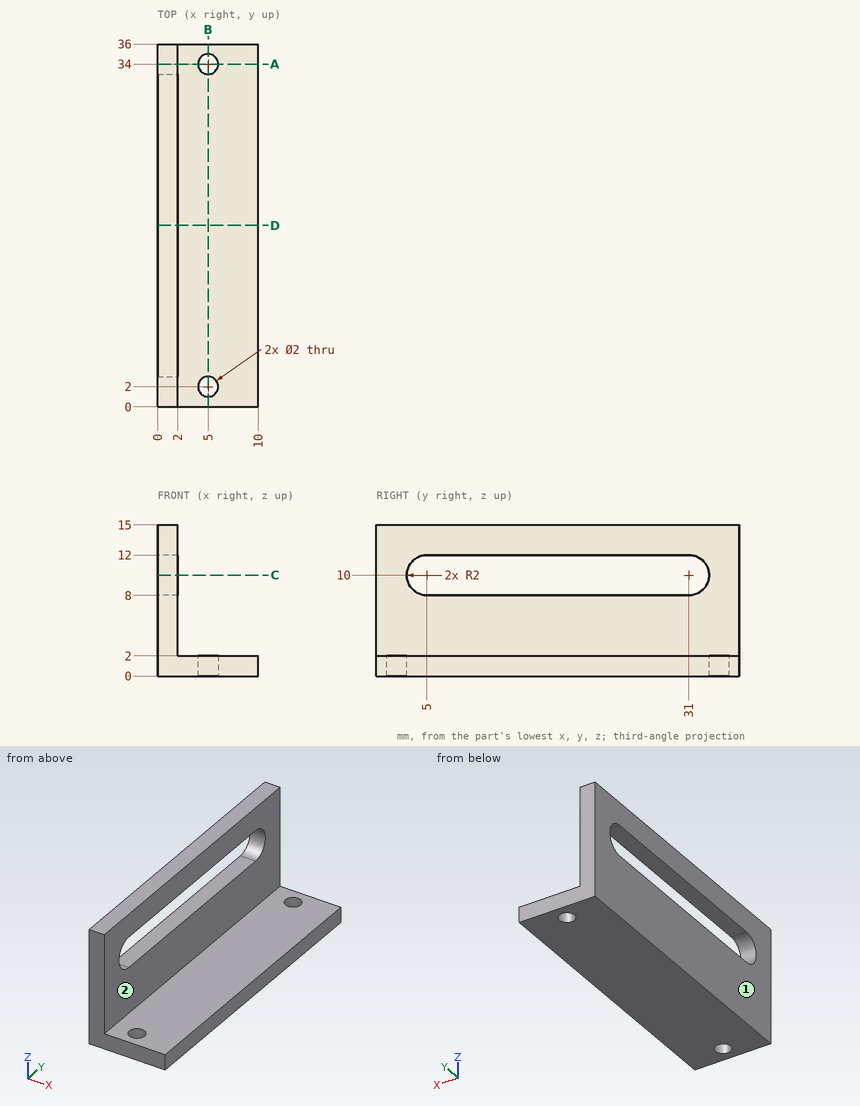
Study the drawing (mm; zero at the part's minimum x, y, z) and answer. A direction names the side the tool comes from. Round coordinates to 2 decimals unless told otherwise and drop trailing zeros. Order: outer loops, then holes, each group sorted by start corner. A loop starts at its lowest first (then second) coordinate and runs counter-clockwise, first axis right, second up. Notation, with made-up numbers: (-8, 26) -> (39, 26) arc R11 cw to (39, 40) -> close; hole circle Ø5 at (80.5, 62.5). An arc over 180 degrees is marked (long way). Answer as CSV lines item,"result". Start each with the question number.
(1) The part is cut by section C-C (z = 10). Determine the outline of the cut face in (x, y), then the cut area to 3 significant figures.
(2) The part is cut by section D-D (y = 18). Determine the outline of the cut face in (x, z).
(3) The part is cut by section A-A (y = 34). Determine the outline of the cut face in (x, z), then the cut area to 3 significant figures.
(4) The part is cut by section B-B (x = 5). Determine the outline of the cut face in (y, z), then the cut area to 3 significant figures.
(5) Flat-ended cylindrical pins translate along their axes: pin 1 Ø1 at (x, y) = (7.5, 20) entering from -Z; pin 2 Ø5 at (x, y) = (5.5, 12) entering from +Z; pin 3 Ø1.5 at (y, z) = (25, 7.5) entering from +X. Find the tip coordinate at first contact, or state that the pin passes through.
(6) A tool of negligible diameter and unlimited length cuts with its end or side. For the marked faces 1 and 2, from which of +Z, -Z, +X, -X, +Y, -Y can it reach the whole face along a straight path? Write none if from no direction.
(7) Find the intervals of material crossed by probe 1 along Y at (x, z) = (5, 1); probe 2 along Z at (x, y) = (1.5, 21); probe 3 along X at (y, z) = (11.5, 14.75), in increasing order. Write a range as from..to.
Evaluation:
1,outline,"(0, 0) -> (2, 0) -> (2, 3) -> (0, 3) -> close; (0, 33) -> (2, 33) -> (2, 36) -> (0, 36) -> close"
1,area,"12.0 mm²"
2,outline,"(0, 0) -> (10, 0) -> (10, 2) -> (2, 2) -> (2, 8) -> (0, 8) -> close; (0, 12) -> (2, 12) -> (2, 15) -> (0, 15) -> close"
3,outline,"(0, 0) -> (4, 0) -> (4, 2) -> (2, 2) -> (2, 15) -> (0, 15) -> close; (6, 0) -> (10, 0) -> (10, 2) -> (6, 2) -> close"
3,area,"42.0 mm²"
4,outline,"(0, 0) -> (1, 0) -> (1, 2) -> (0, 2) -> close; (3, 0) -> (33, 0) -> (33, 2) -> (3, 2) -> close; (35, 0) -> (36, 0) -> (36, 2) -> (35, 2) -> close"
4,area,"64.0 mm²"
5,pin 1,"z = 0"
5,pin 2,"z = 2"
5,pin 3,"x = 2"
6,face 1,"+Z, -Z, -X, +Y, -Y"
6,face 2,"+Z, +X, +Y, -Y"
7,probe 1,"0..1, 3..33, 35..36"
7,probe 2,"0..8, 12..15"
7,probe 3,"0..2"
